Geometry: final body of the model. Coordinates: model frame, mm. Face numbers are marked on the shaded views. A direction names the side the tool comes from. Round coordinates to 2 decimals unless told otherwise and drop trailing zeros. Loops run counter-clockwise (first coordinate to the right, second up) from the corner with the lowest first, then second, coordinate; pieces in that order, holes last. Notation, with made-up numbers: (86.25, 74.25) -> (119.25, 74.25) arc R22 ccw to (119.25, 94.25) -> close; hole circle Ø9 at (89, 62.5). An arc over 180 degrees is marked (long way). Answer in a Markdown table with one row per item.
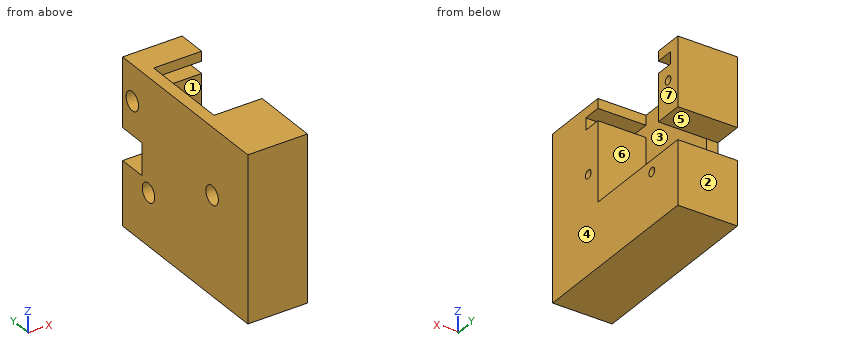
Autodesk Fusion 360 part; units mm, degrees
sketch "Sketch1" plane through (0, 0, 0) normal (1, 0, 0) x (0, 1, 0)
  line L0 (-18.1754, 12.6139) -> (20.3246, 12.6139)
  line L1 (20.3246, 12.6139) -> (20.3246, -16.0861)
  line L2 (20.3246, -16.0861) -> (-18.1754, -16.0861)
  line L3 (-18.1754, -16.0861) -> (-18.1754, 12.6139)
  line L4 (20.3246, -10.1861) -> (12.7246, -10.1861)
  line L5 (12.7246, -10.1861) -> (12.7246, -1.8861)
  line L6 (12.7246, -1.8861) -> (20.3246, -1.8861)
  line L7 (20.3246, -1.8861) -> (20.3246, -10.1861)
  circle A0 centre (16.4746, 1.8639) radius 1.1
  circle A1 centre (-14.3254, -6.0861) radius 1.1
  dimension "d2" = 38.5
  dimension "d3" = 28.7
  dimension "d4" = 7.6
  dimension "d5" = 8.3
  dimension "d6" = 5.9
  dimension "d7" = 2.2
  dimension "d8" = 3.75
  dimension "d9" = 3.85
  dimension "d10" = 2.2
  dimension "d11" = 10
  dimension "d12" = 3.85
extrude "Extrude1" add sketch "Sketch1" along normal blind 15.402 contours L0 L1 L2 L3 L4 L5 L6
sketch "Sketch2" plane through (15.402, 0, 0) normal (1, 0, 0) x (0, 1, 0)
  circle A0 centre (-14.3254, -6.0861) radius 1.1
  circle A1 centre (16.4746, 1.8639) radius 1.1
  line L0 (20.3246, -10.1861) -> (12.7246, -10.1861)
  line L1 (12.7246, -10.1861) -> (12.7246, -1.8861)
  line L2 (12.7246, -1.8861) -> (20.3246, -1.8861)
  line L3 (20.3246, -1.8861) -> (20.3246, 12.6139)
  line L4 (20.3246, 12.6139) -> (-18.1754, 12.6139)
  line L5 (-18.1754, 12.6139) -> (-18.1754, -16.0861)
  line L6 (-18.1754, -16.0861) -> (20.3246, -16.0861)
  line L7 (20.3246, -16.0861) -> (20.3246, -10.1861)
  line L8 (12.7246, -10.1861) -> (-10.5754, -10.1861)
  line L9 (-10.5754, -10.1861) -> (-10.5754, 12.6139)
  line L10 (-10.5754, 12.6139) -> (12.7246, 12.6139)
  line L11 (12.7246, 12.6139) -> (12.7246, -10.1861)
  line L12 (12.7246, 8.6139) -> (17.4246, 8.6139)
  line L13 (17.4246, 8.6139) -> (17.4246, 5.5139)
  line L14 (17.4246, 5.5139) -> (12.7246, 5.5139)
  line L15 (12.7246, 5.5139) -> (12.7246, 8.6139)
  line L16 (-10.5754, 5.5139) -> (-15.2754, 5.5139)
  line L17 (-15.2754, 5.5139) -> (-15.2754, 8.6139)
  line L18 (-15.2754, 8.6139) -> (-10.5754, 8.6139)
  line L19 (-10.5754, 8.6139) -> (-10.5754, 5.5139)
  dimension "d15" = 23.3
  dimension "d16" = 4.7
  dimension "d17" = 3.1
  dimension "d18" = 21.6
  dimension "d19" = 4.7
  dimension "d20" = 3.1
  dimension "d21" = 21.6
extrude "Extrude2" cut sketch "Sketch2" against normal blind 12.402 contours L1 L4 L8 L9 L10 L11 L15 L19 | L11 L12 L13 L14 L15 | L9 L16 L17 L18 L19
sketch "Sketch3" plane through (0, 0, 0) normal (-1, 0, 0) x (0, -1, 0)
  circle A0 centre (14.3254, -6.0861) radius 1.1
  circle A1 centre (-16.4746, 1.8639) radius 1.1
  line L0 (-12.7246, -10.1861) -> (-20.3246, -10.1861)
  line L1 (-20.3246, -10.1861) -> (-20.3246, -16.0861)
  line L2 (-20.3246, -16.0861) -> (18.1754, -16.0861)
  line L3 (18.1754, -16.0861) -> (18.1754, 12.6139)
  line L4 (18.1754, 12.6139) -> (-20.3246, 12.6139)
  line L5 (-20.3246, 12.6139) -> (-20.3246, -1.8861)
  line L6 (-20.3246, -1.8861) -> (-12.7246, -1.8861)
  line L7 (-12.7246, -1.8861) -> (-12.7246, -10.1861)
  circle A2 centre (-16.4746, 1.8639) radius 2.4
  circle A3 centre (14.3254, -6.0861) radius 2.4
  dimension "d24" = 4.8
  dimension "d25" = 4.8
extrude "Extrude3" cut sketch "Sketch3" against normal blind 7.701 contours A2
extrude "Extrude4" cut sketch "Sketch3" against normal blind 7.701 contours A3
extrude "Extrude5" cut 1 faces at (11.268, 7.4913, -10.1861) along direction (0, 0, -1) blind 4.8
extrude "Extrude6" add 1 faces at (5.134, 7.4913, -16.0861) along direction (0, 0, -1) blind 5
extrude "Extrude7" cut 1 faces at (5.134, 7.4913, -21.0861) along direction (0, 0, 1) blind 0.1
extrude "Extrude8" cut 1 faces at (5.134, -18.1754, 1.4139) along direction (0, 1, 0) blind 0.1
extrude "Extrude9" cut 1 faces at (5.134, 20.3246, 7.7806) along direction (0, -1, 0) blind 0.1
extrude "Extrude10" cut 1 faces at (5.134, 20.3246, -18.9861) along direction (0, -1, 0) blind 0.1
extrude "Extrude11" cut 1 faces at (6.134, 17.7246, 12.6139) along direction (0, 0, -1) blind 1
extrude "Extrude12" cut 1 faces at (6.134, 17.7246, 11.6139) along direction (0, 0, -1) blind 0.5
sketch "Sketch4" plane through (15.402, 0, 0) normal (1, 0, 0) x (0, 1, 0)
  line L0 (-10.5754, 11.1139) -> (-18.0754, 11.1139)
  line L1 (-18.0754, 11.1139) -> (-18.0754, -20.9861)
  line L2 (-18.0754, -20.9861) -> (20.2246, -20.9861)
  line L3 (20.2246, -20.9861) -> (20.2246, -14.9861)
  line L4 (20.2246, -14.9861) -> (-10.5754, -14.9861)
  line L5 (-10.5754, -14.9861) -> (-10.5754, 5.5139)
  line L6 (-10.5754, 5.5139) -> (-15.2754, 5.5139)
  line L7 (-15.2754, 5.5139) -> (-15.2754, 8.6139)
  line L8 (-15.2754, 8.6139) -> (-10.5754, 8.6139)
  line L9 (-10.5754, 8.6139) -> (-10.5754, 11.1139)
  circle A0 centre (-14.3254, -6.0861) radius 1.1
  circle A1 centre (10.2246, -18) radius 1.1
  dimension "d46" = 2.2
  dimension "d72" = 10
extrude "Extrude13" cut sketch "Sketch4" against normal blind 15.402 contours A1
sketch "Sketch5" plane through (0, 0, 0) normal (-1, 0, 0) x (0, -1, 0)
  circle A0 centre (-10.2246, -18) radius 1.1
  line L0 (18.0754, 11.1139) -> (-20.2246, 11.1139)
  line L1 (-20.2246, 11.1139) -> (-20.2246, -1.8861)
  line L2 (-20.2246, -1.8861) -> (-12.7246, -1.8861)
  line L3 (-12.7246, -1.8861) -> (-12.7246, -14.9861)
  line L4 (-12.7246, -14.9861) -> (-20.2246, -14.9861)
  line L5 (-20.2246, -14.9861) -> (-20.2246, -20.9861)
  line L6 (-20.2246, -20.9861) -> (18.0754, -20.9861)
  line L7 (18.0754, -20.9861) -> (18.0754, 11.1139)
  circle A1 centre (14.3254, -6.0861) radius 2.4
  circle A2 centre (-16.4746, 1.8639) radius 2.4
  circle A3 centre (-10.2246, -18) radius 2.4
  dimension "d49" = 4.8
extrude "Extrude14" cut sketch "Sketch5" against normal blind 7.701 contours A3
extrude "Extrude15" add 1 faces at (6.134, 17.7246, -1.8861) along direction (0, 0, -1) blind 4.8
extrude "Extrude16" add 1 faces at (5.134, 7.4579, -20.9861) along direction (0, 0, -1) blind 0.5
extrude "Extrude17" add 1 faces at (5.134, 7.4579, -21.4861) along direction (0, 0, -1) blind 10
extrude "Extrude18" add 1 faces at (5.134, -18.0754, -3.0861) along direction (0, -1, 0) blind 10
Item 1: First-contact query: P1, Ø4.5, axis at y = 16.47, z = 1.86, coming from the +X side; P2, Ø13, axis at y = 6, z = 3, coming from the +X side; P3, Ø3.5, axis at x = 1.5, z = -9.5, coming from the +Y side; P4, Ø2.5, axis at y = 9.5, z = -17.5, coming from the -X side. Flat tips, straight axial feed; report the tip coordinate or a pass-through.
Ans:
| item | result |
|---|---|
| P1 | x = 15.4 |
| P2 | x = 3 |
| P3 | y = 12.72 |
| P4 | x = 7.7 |
Item 2: Set-up query: the marked faces 5, 6 and 7. Return all of +Z, -Z, +X, -X, +Y, -Y with unobstructed straight access to the full face (end or side cutting, diameter ignored); none if empty.
Ans:
| item | result |
|---|---|
| face 5 | +X, -X, +Y |
| face 6 | +Z, +X |
| face 7 | +Z, -Z, +X, +Y, -Y |
Item 3: Section query B-B, the plane z = -18. Output: boundary loops of the cut face in (x, y), and give its area (3 significant figures).
Ans:
| item | result |
|---|---|
| outline | (0, -28.08) -> (15.4, -28.08) -> (15.4, 9.12) -> (7.7, 9.12) -> (7.7, 7.82) -> (0, 7.82) -> close; (0, 12.62) -> (7.7, 12.62) -> (7.7, 11.32) -> (15.4, 11.32) -> (15.4, 20.22) -> (0, 20.22) -> close |
| area | 690 mm2 |
Item 4: Section query A-A, the plane x = 14.25. Output: boundary loops of the cut face in (y, z), and give its area (3 significant figures).
Ans:
| item | result |
|---|---|
| outline | (-28.08, -31.49) -> (20.22, -31.49) -> (20.22, -14.99) -> (-10.58, -14.99) -> (-10.58, 5.51) -> (-15.28, 5.51) -> (-15.28, 8.61) -> (-10.58, 8.61) -> (-10.58, 11.11) -> (-28.08, 11.11) -> close; (12.72, -6.69) -> (20.22, -6.69) -> (20.22, 11.11) -> (12.72, 11.11) -> (12.72, 8.61) -> (17.42, 8.61) -> (17.42, 5.51) -> (12.72, 5.51) -> close; hole circle Ø2.2 at (-14.33, -6.09); hole circle Ø2.2 at (10.22, -18); hole circle Ø2.2 at (16.47, 1.86) |
| area | 1,350 mm2 |
Item 5: Ray query, L1, parallel to Z at x = 15, y = 15; L2, parallel to Z at x = 11, y = -11; L3, parallel to Y at x = 10.75, z = 7. Return the intervals inside material, ascending.
Ans:
| item | result |
|---|---|
| L1 | -31.49 to -14.99, -6.69 to 5.51, 8.61 to 11.11 |
| L2 | -31.49 to 5.51, 8.61 to 11.11 |
| L3 | -28.08 to -15.28, 17.42 to 20.22 |
Item 6: Mould query, pull axis Y, two halves, no side actions, for the marked faces 1, 2, 3 and 4. Classes: released by +Y, released by -Y, zero draft, split by the parting line, or undercut.
Ans:
| item | result |
|---|---|
| face 1 | undercut |
| face 2 | released by +Y |
| face 3 | undercut |
| face 4 | zero draft |
Item 7: Section query D-D, the plane z = -9.5. Output: boundary loops of the cut face in (x, y), and give its area (3 significant figures).
Ans:
| item | result |
|---|---|
| outline | (0, -28.08) -> (15.4, -28.08) -> (15.4, -10.58) -> (3, -10.58) -> (3, 12.72) -> (0, 12.72) -> close |
| area | 339 mm2 |
Item 8: Section query C-C, the plane y = 6.5. Output: boundary loops of the cut face in (x, z), and give its area (3 significant figures).
Ans:
| item | result |
|---|---|
| outline | (0, -31.49) -> (15.4, -31.49) -> (15.4, -14.99) -> (3, -14.99) -> (3, 11.11) -> (0, 11.11) -> close |
| area | 332 mm2 |
